Solid Edge part; units mm, degrees
sketch "Sketch1" plane through (0, 0, 0) normal (0, 0, 1) x (1, 0, 0)
  circle A0 centre (0, 0) radius 1.5
extrude "Protrusion1" add sketch "Sketch1" along normal blind 5
sketch "Sketch2" plane through (0, 0, 5) normal (0, 0, 1) x (1, 0, 0)
  line L0 (2.25, 1.299) -> (0, 2.5981)
  line L1 (0, 2.5981) -> (-2.25, 1.299)
  line L2 (-2.25, 1.299) -> (-2.25, -1.299)
  line L3 (-2.25, -1.299) -> (0, -2.5981)
  line L4 (0, -2.5981) -> (2.25, -1.299)
  line L5 (2.25, -1.299) -> (2.25, 1.299)
extrude "ExtrudedProtrusion_2" add sketch "Sketch2" along normal blind 5
sketch "Sketch3" plane through (0, 0, 10) normal (0, 0, 1) x (0, 1, 0)
  circle A0 centre (0, 0) radius 1.5
extrude "ExtrudedCutout_1" cut sketch "Sketch3" against normal blind 4.5
fillet "Round_1" radius 0.2 20 edges at (2.25, -1.299, 7.5) (2.25, 1.299, 7.5) (2.25, 0, 10) (1.125, 1.9486, 10) (0, -1.5, 10) (0, 2.5981, 7.5) (1.125, 1.9486, 5) (2.25, 0, 5) (1.125, -1.9486, 5) (0, -2.5981, 7.5) (1.125, -1.9486, 10) (-1.125, -1.9486, 10) (-1.125, -1.9486, 5) (-2.25, -1.299, 7.5) (-2.25, 0, 10) (-1.125, 1.9486, 10) (-2.25, 1.299, 7.5) (-2.25, 0, 5) (-1.125, 1.9486, 5) (-1.5, 0, 0)
properties material "Brass, yellow brass"
For this review, take the finished solid that the model builds, in its own axes (mm). A direction names the side the tool comes from. Round coordinates to 2 decimals unless told otherwise and drop trailing zeros. Write each loop counter-clockwise with the first axis right and the second up, starting at its lowest first coordinate (ties: lowest second). Pieces come first, ordered by that corner, then holes. Notation, with made-up numbers: (-37.75, 2) -> (4.25, 2) arc R24 ccw to (4.25, 30) -> close; hole circle Ø1 at (-22.5, 59). An arc over 180 degrees is marked (long way). Use one line per item in the form item = value.
Q1. Clearance check with flat-ended pins moving along their axes: pin 1 Ø2.5 at (x, y) = (0, 0) entering from +Z; pin 2 Ø2 at (x, z) = (-1.5, 5.5) entering from +Y; pin 3 Ø1 at (y, z) = (-2, 9) entering from -X. State where each tip first meets the part, or that it passes through.
Resolved:
pin_1 = 5.5
pin_2 = 2.31
pin_3 = -1.9
Q2. Machinability: for faces 4 (the flat face through (0, -2, 5)), 5 (the cylindrical face through (-0.07, -1.5, 7.68)), 6 (the flat face through (-1.14, -1.94, 7.47)), which of the approach directions +Z, -Z, +X, -X, +Y, -Y give a long, thin tool a straight path to every point of the face, cutting with its end or side? Answer none if there is none.
Resolved:
face_4 = -Z
face_5 = +Z
face_6 = +Z, -Z, -X, -Y
Q3. The part is to be moulded in two halves that separate along Y. For faces 1 (the flat face through (0, 0, 5.5)), 2 (the flat face through (2.25, 0, 7)), 3 (the cylindrical face through (1.08, 1.91, 5.06)), say which applies: released by +Y, released by -Y, zero draft, split by the parting line, or undercut.
Resolved:
face_1 = undercut
face_2 = zero draft
face_3 = released by +Y
Q4. To check wall thickness, follow probe 1 along Y at (x, z) = (0, 8.55); probe 2 along X at (y, z) = (0, 7.75); probe 3 along Z at (x, y) = (-1.5, 1.05). State the ranges of each line that lie inside material, in increasing order. Write a range as from..to.
Resolved:
probe_1 = -2.57..-1.5, 1.5..2.57
probe_2 = -2.25..-1.5, 1.5..2.25
probe_3 = 5..10
Q5. Consider section C-C (z = 1). State the section outline as (x, y) points, then the cut area to 3 significant figures.
Resolved:
outline = circle Ø3 at (0, 0)
area = 7.07 mm²
Q6. Consider section A-A (z = 7.5). State the section outline as (x, y) points, then the cut area to 3 significant figures.
Resolved:
outline = (-2.25, -1.18) arc R0.2 ccw to (-2.15, -1.36) -> (-0.1, -2.54) arc R0.2 ccw to (0.1, -2.54) -> (2.15, -1.36) arc R0.2 ccw to (2.25, -1.18) -> (2.25, 1.18) arc R0.2 ccw to (2.15, 1.36) -> (0.1, 2.54) arc R0.2 ccw to (-0.1, 2.54) -> (-2.15, 1.36) arc R0.2 ccw to (-2.25, 1.18) -> close; hole circle Ø3 at (0, 0)
area = 10.5 mm²
Q7. Consider section B-B (y = 0). State the section outline as (x, z) points.
Resolved:
outline = (-2.25, 5.2) arc R0.2 ccw to (-2.05, 5) -> (-1.5, 5) -> (-1.5, 0.2) arc R0.2 ccw to (-1.3, 0) -> (1.3, 0) arc R0.2 ccw to (1.5, 0.2) -> (1.5, 5) -> (2.05, 5) arc R0.2 ccw to (2.25, 5.2) -> (2.25, 9.8) arc R0.2 ccw to (2.05, 10) -> (1.7, 10) arc R0.2 ccw to (1.5, 9.8) -> (1.5, 5.5) -> (-1.5, 5.5) -> (-1.5, 9.8) arc R0.2 ccw to (-1.7, 10) -> (-2.05, 10) arc R0.2 ccw to (-2.25, 9.8) -> close
